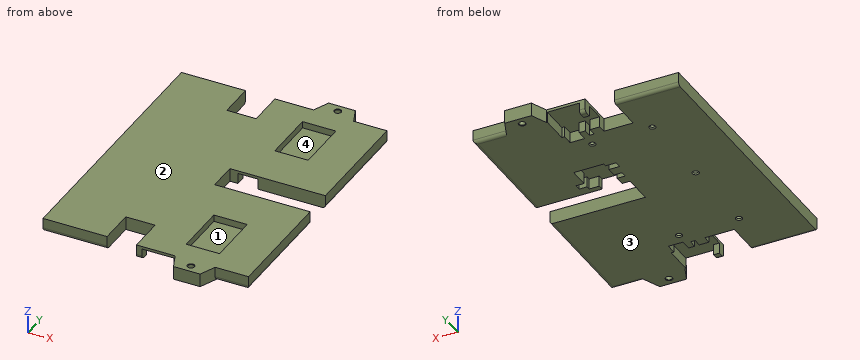
Solid Edge part; units mm, degrees
sketch "Sketch1" plane through (0, 0, 0) normal (0, -1, 0) x (1, 0, 0)
  line L0 (-175, -5) -> (175, -5)
  line L1 (175, -5) -> (175, 5)
  line L2 (175, 5) -> (-175, 5)
  line L3 (-175, 5) -> (-175, -5)
  dimension "D1" = 175
  dimension "D2" = 175
extrude "Protrusion1" add sketch "Sketch1" against normal blind 200
sketch "Sketch2" plane through (0, 100, -5) normal (0, 0, -1) x (1, 0, 0)
  line L0 (-21.8, 78.97) -> (-21.8, 72.97)
  line L1 (-21.8, 72.97) -> (-18.3, 72.97)
  line L2 (-18.3, 72.97) -> (-18.3, 78.97)
  line L3 (-18.3, 78.97) -> (-15.3, 78.97)
  line L4 (-15.3, 78.97) -> (-10.3, 78.97)
  line L5 (-10.3, 78.97) -> (-10.3, 93.97)
  line L6 (-10.3, 93.97) -> (-15.3, 93.97)
  line L7 (-15.3, 93.97) -> (-15.3, 101.97)
  line L8 (-15.3, 101.97) -> (-18.3, 101.97)
  line L9 (-18.3, 101.97) -> (-18.3, 107.97)
  line L10 (-18.3, 107.97) -> (-21.8, 107.97)
  line L11 (-21.8, 107.97) -> (-21.8, 101.97)
  line L12 (-21.8, 101.97) -> (-39.3, 101.97)
  line L13 (-39.3, 101.97) -> (-39.3, 78.97)
  line L14 (-39.3, 78.97) -> (-37.3, 78.97)
  line L15 (-37.3, 78.97) -> (-37.3, 70.97)
  line L16 (-37.3, 70.97) -> (-26.3, 70.97)
  line L17 (-26.3, 70.97) -> (-26.3, 78.97)
  line L18 (-26.3, 78.97) -> (-21.8, 78.97)
  dimension "D1" = 39.3
  dimension "D2" = 21.8
  dimension "D3" = 18.3
  dimension "D4" = 15.3
  dimension "D5" = 10.3
  dimension "D6" = 37.3
  dimension "D7" = 37.3
extrude "Cutout1" cut sketch "Sketch2" against normal blind 8
sketch "Sketch3" plane through (0, 100, -5) normal (0, 0, -1) x (1, 0, 0)
  line L0 (11, 72.97) -> (-11, 72.97)
  line L1 (-11, 111.97) -> (-11, 72.97)
  line L2 (11, 111.97) -> (-11, 111.97)
  line L3 (11, 111.97) -> (11, 72.97)
  dimension "D1" = 11
  dimension "D2" = 11
extrude "Cutout2" cut sketch "Sketch3" against normal through all
mirror "Mirror1" about plane through (0, 100, 0) normal (0, -1, 0) of "Cutout1", "Cutout2"
mirror "Mirror2" about plane through (40, 0, 0) normal (1, 0, 0) of "Mirror1", "Cutout2", "Cutout1"
mirror "Mirror3" about plane through (-40, 0, 0) normal (1, 0, 0) of "Cutout2", "Cutout1", "Mirror1"
sketch "Sketch4" plane through (0, 100, -5) normal (0, 0, -1) x (0, -1, 0)
  line L0 (-22.6, 109.45) -> (-22.6, 103.45)
  line L1 (-22.6, 103.45) -> (-18.1, 103.45)
  line L2 (-18.1, 103.45) -> (-18.1, 109.45)
  line L3 (-18.1, 109.45) -> (-15.1, 109.45)
  line L4 (-15.1, 109.45) -> (-11, 109.45)
  line L5 (-11, 109.45) -> (-11, 124.45)
  line L6 (-11, 124.45) -> (-15.1, 124.45)
  line L7 (-15.1, 124.45) -> (-15.1, 131.95)
  line L8 (-15.1, 131.95) -> (-18.1, 131.95)
  line L9 (-18.1, 131.95) -> (-18.1, 137.95)
  line L10 (-18.1, 137.95) -> (-22.6, 137.95)
  line L11 (-22.6, 137.95) -> (-22.6, 131.95)
  line L12 (-22.6, 131.95) -> (-37.6, 131.95)
  line L13 (-37.6, 131.95) -> (-37.6, 109.45)
  line L14 (-37.6, 109.45) -> (-35.1, 109.45)
  line L15 (-35.1, 109.45) -> (-35.1, 101.45)
  line L16 (-35.1, 101.45) -> (-30.1, 101.45)
  line L17 (-30.1, 101.45) -> (-30.1, 109.45)
  line L18 (-30.1, 109.45) -> (-22.6, 109.45)
  dimension "D1" = 22.6
  dimension "D2" = 18.1
  dimension "D3" = 15.1
  dimension "D4" = 11
  dimension "D5" = 37.6
  dimension "D6" = 35.1
  dimension "D7" = 35.1
  dimension "D8" = 37.6
  dimension "D9" = 22.6
extrude "Cutout3" cut sketch "Sketch4" against normal up to vertex (8 mm away)
sketch "Sketch5" plane through (0, 100, -5) normal (0, 0, -1) x (0, -1, 0)
  line L0 (-11, 109.45) -> (-11, 103.45)
  line L1 (-11, 103.45) -> (11, 103.45)
  line L2 (11, 103.45) -> (11, 175)
  line L3 (11, 175) -> (-11, 175)
  line L4 (-11, 175) -> (-11, 109.45)
  dimension "D1" = 11
  dimension "D2" = 11
extrude "Cutout4" cut sketch "Sketch5" against normal through all
mirror "Mirror4" about plane through (0, 0, 0) normal (1, 0, 0) of "Cutout4", "Cutout3"
sketch "Sketch6" plane through (0, 100, -5) normal (0, 0, -1) x (1, 0, 0)
  circle A0 centre (-97.5, 62.5) radius 1.875
  circle A1 centre (-52.5, 62.5) radius 1.875
  circle A2 centre (-52.5, 0) radius 1.875
  circle A3 centre (-97.5, -62.5) radius 1.875
  circle A4 centre (-52.5, -62.5) radius 1.875
  dimension "D1" = 97.5
  dimension "D2" = 97.5
extrude "Cutout5" cut sketch "Sketch6" against normal blind 7
sketch "Sketch7" plane through (0, 100, 5) normal (0, 0, 1) x (1, 0, 0)
  line L0 (-120, 84) -> (-120, 44)
  line L1 (-120, 44) -> (-145, 44)
  line L2 (-145, 44) -> (-145, 84)
  line L3 (-145, 84) -> (-120, 84)
  dimension "D1" = 145
  dimension "D2" = 145
extrude "Cutout6" cut sketch "Sketch7" against normal blind 5
mirror "Mirror5" about plane through (0, 100, 0) normal (0, -1, 0) of "Cutout6"
mirror "Mirror6" about plane through (0, 0, 0) normal (1, 0, 0) of "Cutout6", "Mirror5"
sketch "Sketch8" plane through (0, 100, 5) normal (0, 0, 1) x (1, 0, 0)
  line L0 (21, 100) -> (21, -100)
extrude "Cutout7" cut sketch "Sketch8" against normal through all material side at (20.95, 100, 5)
hole "Hole_11" at (105, 37.5, -5) direction (0, 0, 1) diameter 3.7 depth 5 tip angle 118 start chamfer 0.6 start chamfer angle 30 end chamfer 0.6 end chamfer angle 30
hole "Hole1" at (105, 162.5, -5) direction (0, 0, 1) diameter 3.7 depth 5 tip angle 118 start chamfer 0.6 start chamfer angle 30 end chamfer 0.6 end chamfer angle 30
hole "Hole2" at (60, 37.5, -5) direction (0, 0, 1) diameter 3.7 depth 5 tip angle 118 start chamfer 0.6 start chamfer angle 30 end chamfer 0.6 end chamfer angle 30
hole "Hole3" at (60, 100, -5) direction (0, 0, 1) diameter 3.7 depth 5 tip angle 118 start chamfer 0.6 start chamfer angle 30 end chamfer 0.6 end chamfer angle 30
hole "Hole4" at (60, 162.5, -5) direction (0, 0, 1) diameter 3.7 depth 5 tip angle 118 start chamfer 0.6 start chamfer angle 30 end chamfer 0.6 end chamfer angle 30
sketch "Sketch9" plane through (98, 100, -5) normal (0, 0, -1) x (1, 0, 0)
  line L0 (22, 100) -> (27, 112)
  line L1 (27, 112) -> (47, 112)
  line L2 (47, 112) -> (52, 100)
  line L3 (52, 100) -> (22, 100)
  dimension "D1" = 52
  dimension "D2" = 27
  dimension "D3" = 47
extrude "Protrusion2" add sketch "Sketch9" against normal up to vertex (10 mm away)
hole "Hole_16" at (135, -6, -5) direction (0, 0, 1) diameter 4.5 end up to next start chamfer 0.4 start chamfer angle 45 end chamfer 0.4 end chamfer angle 45
mirror "Mirror7" about plane through (0, 100, 0) normal (0, -1, 0) of "Protrusion2", "Hole_16"
fillet "Round1" radius 2.5 8 edges at (45, 200, -5) (93.15, 200, -5) (162.5, 200, -5) (175, 155.5, -5) (175, 44.5, -5) (162.5, 0, -5) (93.15, 0, -5) (45, 0, -5)
properties material "Nylon, allgemein"
The model under review builds one solid part; all positions refer to its coordinate system, in mm. Face numbers are marked on the shaded views. A direction names the side the tool comes from. Give positions to 0.01 mm unless a question says otherwise; leave off trailing zeros. Loops run counter-clockwise (first coordinate to the right, second up) from the corner with the lowest first, then second, coordinate; pieces in that order, holes last. Notation, with made-up numbers: (11.5, 11) - (67.5, 11) arc R28 ccw to (67.5, 34) - close; hole circle Ø5 at (55, 54.5). An arc over 180 degrees is marked (long way). Answer as a JSON object with one key per item and string values.
Q1. To check wall thickness, follow line 1 along Y through (x, z) = (60, -0.9); line 2 along X through (y, z) = (199, 1.5); line 3 along Y through (x, z) = (105, -3). State the ranges of each line that lie inside material, in increasing order.
Worked out:
{"line 1": "y = 0 to 35.65, 39.35 to 98.15, 101.85 to 160.65, 164.35 to 200", "line 2": "x = 21 to 69, 91 to 95.3, 119.3 to 175", "line 3": "y = 21.03 to 35.65, 39.35 to 89, 111 to 118.1, 122.6 to 130.1, 135.1 to 160.65, 164.35 to 178.97"}
Q2. For the marked faces 3 and 4, list the 3-axis set-ups (+Z, -Z, +X, -X, +Y, -Y) from which the entire face can be reached by the end or side of a thin tool; tool diameter is ignored.
Worked out:
{"face 3": "-Z, +X, -X, +Y, -Y", "face 4": "+Z"}
Q3. Insertion check: pin 1 (5 mm diameter, centred on x = 80.5, z = 1.5, fed in from -Y); pin 2 (5 mm diameter, centred on x = 103, z = -2, fed in from -Y). Each pin has a flat end and moves straight along its axis. Give the tip position at first contact, or say it passes through.
Worked out:
{"pin 1": "stops at y = 27.03", "pin 2": "stops at y = 21.03"}
Q4. Add section B-B on x = 135. Count the separate pieces of the cut face and the enclosed holes in it, plus the area to 3 significant figures.
Worked out:
{"separate pieces": "4", "enclosed holes": "0", "area": "1,490 mm^2"}
Q5. Mouldability with a two-part tool opening along Y and no side actions: class the marked faces 1 and 2 as +Y half, -Y half, draft (parallel to the pull), parting line (faces both ways), or undercut.
Worked out:
{"face 1": "undercut", "face 2": "draft"}
Q6. Add section C-C on x = 80. State the section outline as (y, z) points, plus the area to 3 significant figures.
Worked out:
{"outline": "(27.03, -5) - (172.97, -5) - (172.97, 5) - (27.03, 5) - close", "area": "1,460 mm^2"}
Q7. Add section A-A on y = -6. State the section outline as (x, z) points.
Worked out:
{"outline": "(122.5, -5) - (132.35, -5) - (132.75, -4.6) - (132.75, 4.6) - (132.35, 5) - (122.5, 5) - close; (137.25, -4.6) - (137.65, -5) - (147.5, -5) - (147.5, 5) - (137.65, 5) - (137.25, 4.6) - close"}
